For this review, take the finished solid that the model builds, in its own axes (mm). Face numbers are marked on the shaded views. A direction names the side the tool comes from. Give positions to 0.01 mm unless a question says otherwise; leave off trailing zeros. Loops run counter-clockwise (first coordinate to the right, second up) from the corner with the lowest first, then second, coordinate; pieces in that order, holes last. Notation, with made-up numbers: (23.25, -0.5) - (61.25, -0.5) arc R24 cw to (61.25, 23.5) - close; hole circle Ø6 at (39.25, 26.25). An arc over 180 degrees is marked (long way). Answer as CSV lines item,"result".
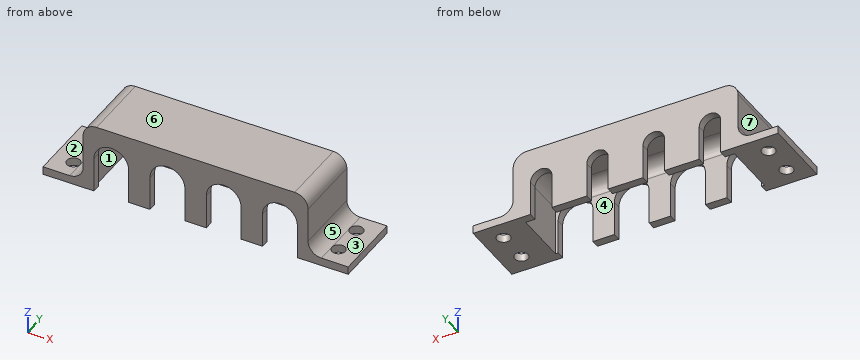
from build123d import *

# Parameters (mm, degrees)
F1_W          = 84
F1_H          = 26
F2_DEPTH      = 13
F2_DEPTH_BACK = 13
F3_T          = -3
F5_W          = 15
F5_H          = 26
F5_R          = 2.5
F5_W_2        = 84
F5_W_3        = 78
F5_H_2        = 20
F6_DEPTH      = 3
F7_R          = 4.99999
F9_DEPTH      = 5
F10_DEPTH     = 25


# Not quite as in the source:
# - a fillet or chamfer is up to 0.001 mm smaller than in the source, because OpenCascade refuses the exact size


with BuildPart() as f2:
    # F1 (on Top) → F2 (new body, two sides)
    with BuildSketch(Plane.XY) as f2_sk:
        with Locations((0, 13)):
            Rectangle(F1_W, F1_H)
    extrude(amount=F2_DEPTH)
    extrude(f2_sk.sketch, amount=-F2_DEPTH_BACK)

    # F3
    f3_openings = [f2.faces().sort_by_distance(p)[0] for p in [
        (0, 13, -13),
    ]]
    offset(amount=F3_T, openings=f3_openings)

    # F5 (on face) → F6 (join)
    with BuildSketch(Plane(origin=(0, 0, -13), x_dir=(1, 0, 0), z_dir=(0, 0, -1))):
        with Locations((-49.5, -13)):
            Rectangle(F5_W, F5_H)
        with Locations((-49.5, -19)):
            Circle(F5_R, mode=Mode.SUBTRACT)
        with Locations((-49.5, -7)):
            Circle(F5_R, mode=Mode.SUBTRACT)
        with Locations((0, -13)):
            Rectangle(F5_W_2, F5_H)
        with Locations((0, -13)):
            Rectangle(F5_W_3, F5_H_2, mode=Mode.SUBTRACT)
        with Locations((49.5, -13)):
            Rectangle(F5_W, F5_H)
        with Locations((49.5, -19)):
            Circle(F5_R, mode=Mode.SUBTRACT)
        with Locations((49.5, -7)):
            Circle(F5_R, mode=Mode.SUBTRACT)
    extrude(amount=-F6_DEPTH)

    # F7 (radius 5 in the source; OpenCascade refuses exactly that, so slightly less here)
    f7_edges = [f2.edges().sort_by_distance(p)[0] for p in [
        (-42, 13, 13),
        (42, 13, 13),
        (-42, 13, -10),
        (42, 13, -10),
        (0, 23, 10),
        (0, 3, 10),
        (-39, 13, 10),
        (39, 13, 10),
    ]]
    fillet(f7_edges, radius=F7_R)

    # F8 (on face) → F9 (cut)
    with BuildSketch(Plane.XZ):
        with BuildLine():
            Line((-25, -11), (-25, 0))
            ThreePointArc((-25, 0), (-31.5, 6.5), (-38, 0))
            Line((-38, 0), (-38, -11))
            Line((-38, -11), (-38, -13))
            Line((-38, -13), (-25, -13))
            Line((-25, -13), (-25, -11))
        make_face()
        with BuildLine():
            Line((-4.0000936475, -11), (-4.0000936475, -0.0348913798))
            ThreePointArc((-4.0000936475, -0.0348913798), (-4, 0), (-4.0000936475, 0.0348913798))
            ThreePointArc((-4.0000936475, 0.0348913798), (-10.5909716955, 6.499363365), (-16.9983365331, -0.1470452389))
            Line((-16.9983365331, -0.1470452389), (-16.9983365331, -10.9773843356))
            Line((-16.9983365331, -10.9773843356), (-16.9983365331, -13))
            Line((-16.9983365331, -13), (-4.0000936475, -13))
            Line((-4.0000936475, -13), (-4.0000936475, -11))
        make_face()
        with BuildLine():
            ThreePointArc((4.0000936475, 0.0348913798), (4, 0), (4.0000936475, -0.0348913798))
            Line((4.0000936475, -0.0348913798), (4.0000936475, -11))
            Line((4.0000936475, -11), (4.0000936475, -13))
            Line((4.0000936475, -13), (16.9983365331, -13))
            Line((16.9983365331, -13), (16.9983365331, -10.9773843356))
            Line((16.9983365331, -10.9773843356), (16.9983365331, -0.1470452389))
            ThreePointArc((16.9983365331, -0.1470452389), (10.5909716955, 6.499363365), (4.0000936475, 0.0348913798))
        make_face()
        with BuildLine():
            ThreePointArc((38, 0), (31.5, 6.5), (25, 0))
            Line((25, 0), (25, -11))
            Line((25, -11), (25, -13))
            Line((25, -13), (38, -13))
            Line((38, -13), (38, -11))
            Line((38, -11), (38, 0))
        make_face()
    extrude(amount=-F9_DEPTH, mode=Mode.SUBTRACT)

    # F4 (on face) → F10 (cut)
    with BuildSketch(Plane(origin=(0, 26, 0), x_dir=(-1, 0, 0), z_dir=(0, 1, 0))):
        with BuildLine():
            Line((-6.5, -13), (-6.5, 0))
            ThreePointArc((-6.5, 0), (-10.5, 4), (-14.5, 0))
            Line((-14.5, 0), (-14.5, -13))
            Line((-14.5, -13), (-6.5, -13))
        make_face()
        with BuildLine():
            Line((-27.5, -13), (-27.5, 0))
            ThreePointArc((-27.5, 0), (-31.5, 4), (-35.5, 0))
            Line((-35.5, 0), (-35.5, -13))
            Line((-35.5, -13), (-27.5, -13))
        make_face()
        with BuildLine():
            ThreePointArc((14.5, 0), (10.5, 4), (6.5, 0))
            Line((6.5, 0), (6.5, -13))
            Line((6.5, -13), (14.5, -13))
            Line((14.5, -13), (14.5, 0))
        make_face()
        with BuildLine():
            ThreePointArc((35.5, 0), (31.5, 4), (27.5, 0))
            Line((27.5, 0), (27.5, -13))
            Line((27.5, -13), (35.5, -13))
            Line((35.5, -13), (35.5, 0))
        make_face()
    extrude(amount=-F10_DEPTH, mode=Mode.SUBTRACT)


solid = f2.part
1) Machinability: for the marked faces 1, 2 and 3, which of the approach directions +Z, -Z, +X, -X, +Y, -Y give a long, thin tool a straight path to every point of the face, cutting with its end or side? Answer none if there is none.
From the geometry:
face 1,"-Z"
face 2,"+Z, -X, +Y, -Y"
face 3,"+Z, +X, +Y, -Y"
2) Consider section A-A on x = -49.5. Write out the cut boundary in (y, z).
From the geometry:
outline,"(0, -13) - (4.5, -13) - (4.5, -10) - (0, -10) - close; (9.5, -13) - (16.5, -13) - (16.5, -10) - (9.5, -10) - close; (21.5, -13) - (26, -13) - (26, -10) - (21.5, -10) - close"
3) Wall thickness on line 1 (X direction, y = 7, z = -10.7); line 2 (Y direction, x = 49.5, z = -11.75); line 3 (Y direction, x = -21, z = 4.5): over which ranges is each line inside the solid? List them lowest first. Write a range as from..to.
From the geometry:
line 1,"x = -57..-52, -47..-39, 39..47, 52..57"
line 2,"y = 0..4.5, 9.5..16.5, 21.5..26"
line 3,"y = 0..3, 23..26"
4) Consider section C-C on y = 11.5. Write out the cut boundary in (x, z).
From the geometry:
outline,"(-57, -13) - (-39, -13) - (-39, 5) arc R5 cw to (-34, 10) - (34, 10) arc R5 cw to (39, 5) - (39, -13) - (57, -13) - (57, -10) - (47, -10) arc R5 cw to (42, -5) - (42, 8) arc R5 ccw to (37, 13) - (-37, 13) arc R5 ccw to (-42, 8) - (-42, -5) arc R5 cw to (-47, -10) - (-57, -10) - close"
5) Consider section B-B on y = 19. Count the separate pieces of the cut face and the enclosed holes in it, and give its area (3 significant figures).
From the geometry:
separate pieces,"3"
enclosed holes,"0"
area,"468 mm^2"
6) Consider section D-D on x = -10.5. Write out the cut boundary in (y, z), and give its area (3 significant figures).
From the geometry:
outline,"(0, 6.5) - (3.23, 6.5) arc R5 cw to (8, 10) - (18, 10) arc R5 cw to (23, 5) - (23, 4) - (26, 4) - (26, 13) - (0, 13) - close"
area,"117 mm^2"
7) Draft analysis for pull direction X (two halves, no side actions). For the marked faces 4, 5, 6 and 7, state which applies: pulls with the +X half, pulls with the -X half, needs draft (parallel to the pull), parting line crosses it, or undercut.
From the geometry:
face 4,"undercut"
face 5,"pulls with the +X half"
face 6,"needs draft"
face 7,"pulls with the -X half"
8) Insertion check: P1, Ø3.5, axis at y = 24.5, z = -3.5, coming from the +X side; P2, Ø0.9, axis at y = 25, z = -6, coming from the +X side; P3, Ø11, axis at x = -2, y = 11.5, coming from the -Z side; P4, Ø6.5, axis at x = -49.5, y = 19, coming from the -Z side. Each pin has a flat end and moves straight along its axis. Give the tip position at first contact, or say it passes through.
From the geometry:
P1,"stops at x = 42.01"
P2,"stops at x = 42.21"
P3,"stops at z = 9.58"
P4,"stops at z = -13"
